```python
from build123d import *

# Parameters (mm, degrees)
EXTRUDE_1_DEPTH     = 4
SKETCH_2_R          = 10.75
CUT_EXTRUDE_1_DEPTH = 22.756225163


with BuildPart() as part:
    # 草图1 → 凸台-拉伸1 (new body)
    with BuildSketch(Plane(origin=(0, 0, 0), x_dir=(1, 0, 0), z_dir=(0, 1, 0))):
        Polygon((8.082903769, 14), (-8.082903769, 14), (-16.165807537, 0), (-8.082903769, -14), (8.082903769, -14), (16.165807537, 0), align=None)
    extrude(amount=EXTRUDE_1_DEPTH)

    # 草图2 → 切除-拉伸1 (cut, through all)
    with BuildSketch(Plane(origin=(0, 4, 0), x_dir=(1, 0, 0), z_dir=(0, 1, 0))):
        with Locations(Location((0, 0, 0), (0, 0, 270))):
            Circle(SKETCH_2_R)
    extrude(amount=-CUT_EXTRUDE_1_DEPTH, mode=Mode.SUBTRACT)

    # 草图3 → 切除-旋转1 (revolve, cut)
    with BuildSketch(Plane.XY, mode=Mode.PRIVATE) as cut_revolve_1_sk:
        Polygon((-16.165807537, 4), (-16.165807537, 3.5), (-13.5, 4), align=None)
        Polygon((-13.5, 0), (-16.165807537, 0), (-16.165807537, 0.5), align=None)
    revolve(cut_revolve_1_sk.sketch.rotate(Axis((0, 0, 0), (0, 1, 0)), 270), axis=Axis((0, 0, 0), (0, 1, 0)), mode=Mode.SUBTRACT)


solid = part.part
```
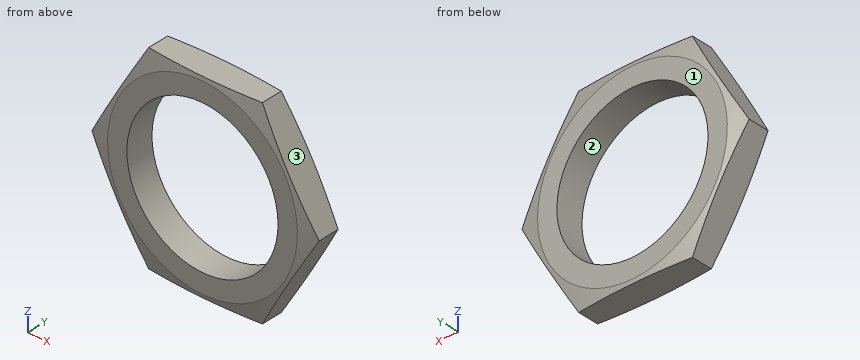
Here's how the part is built. I have some questions about the finished solid (model axes, mm). Face numbers are marked on the shaded views. Coordinates: 2 decimals unless noted, no trailing zeros. Order: outer loops, then holes, each group sorted by start corner. A loop starts at its lowest first (then second) coordinate and runs counter-clockwise, first axis right, second up. Notation, with made-up numbers: M 22,43 L 68,43 A36 ccw 68,82 Z; hole C 72,74.25 d1. An arc over 180 degrees is marked long. Answer as a JSON object with one key per item and string values. Group by question number.
(1) I need wall thicknesses on probe 1 along X at (y, z) = (2.35, 1.75); probe 2 along Z at (x, y) = (0.5, 3.2); probe 3 along X at (y, z) = (2.85, -4.75). Which ranges of each line are inside material? Lowest first, please.
(2) Suppose I cut it at B-B, the plane x = 0. Please give me the cut outline in (y, z), then the cut area to 3 significant figures.
(3) Suppose I cut it at A-A, the plane y = 0.95. Please give me the cut outline in (x, z).
(4) If we mould it in two halves opening along Z, with no side actions, what happens to the marked faces 1, 2 and 3? For each: released by +Z, released by -Z, zero draft, split by the parting line, or undercut.
Values found:
{
 "1": {"probe 1": "x = -15.16 to -10.61, 10.61 to 15.16", "probe 2": "z = -14 to -10.74, 10.74 to 14", "probe 3": "x = -13.42 to -9.64, 9.64 to 13.42"},
 "2": {"outline": "M 0,-13.5 L 0.09,-14 L 3.91,-14 L 4,-13.5 L 4,-10.75 L 0,-10.75 Z; M 0,10.75 L 4,10.75 L 4,13.5 L 3.91,14 L 0.09,14 L 0,13.5 Z", "area": "25.9 mm^2"},
 "3": {"outline": "M -16.17,0 L -8.08,-14 L 8.08,-14 L 16.17,0 L 8.08,14 L -8.08,14 Z; hole C 0,0 d21.5"},
 "4": {"face 1": "zero draft", "face 2": "undercut", "face 3": "released by +Z"}
}
